Geometry check sheet. Reference: the model listing, model coordinates, mm. A direction names the side the tool comes from. Coordinates: 2 decimals unless noted, no trailing zeros. Order: outer loops, then holes, each group sorted by start corner. A loop starts at its lowest first (then second) coordinate and runs counter-clockwise, first axis right, second up. Notation, with made-up numbers: (52.25, -12) -> (87.25, -12) arc R13 ccw to (87.25, -2) -> close; hole circle Ø10 at (89, 63.25). An arc over 180 degrees is marked (long way). Answer as CSV lines item,"result". Start each with the question number.
from build123d import *

# Parameters (mm, degrees)
F0_R     = 8.5
F1_DEPTH = 4
F2_R     = 5
F3_DEPTH = 100


with BuildPart() as f1:
    # F0 (on Top) → F1 (new body)
    with BuildSketch(Plane.XY):
        Circle(F0_R)
    extrude(amount=F1_DEPTH)

    # F2 (on Top) → F3 (join)
    with BuildSketch(Plane.XY):
        Circle(F2_R)
    extrude(amount=F3_DEPTH)

    # F4 (on Right) → F5 (revolve)
    with BuildSketch(Plane.YZ):
        with BuildLine():
            Line((0, 104.582576), (0, 100))
            Line((0, 100), (5, 100))
            ThreePointArc((5, 100), (4.1833, 102.738613), (2, 104.582576))
            Line((2, 104.582576), (0, 104.582576))
        make_face()
    revolve(axis=Axis((0, 0, 104.791288), (0, 0, -1)))

    # F4 (on Right) → F6 (revolve)
    with BuildSketch(Plane.YZ):
        with BuildLine():
            ThreePointArc((0, 105), (1.021548, 104.894532), (2, 104.582576))
            Line((2, 104.582576), (1, 109.582576))
            Line((1, 109.582576), (0, 109.582576))
            Line((0, 109.582576), (0, 105))
        make_face()
        with BuildLine():
            Line((0, 105), (0, 104.582576))
            Line((0, 104.582576), (2, 104.582576))
            ThreePointArc((2, 104.582576), (1.021548, 104.894532), (0, 105))
        make_face()
    revolve(axis=Axis((0, 0, 104.791288), (0, 0, -1)))


solid = f1.part
Q1. Sectioned sample at B-B, the plane x = 6.25. Record the cut outline in (y, z), then the cut area to 3 significant figures.
Q2. Access from +Z, -Z, +X, -X, +Y, -Y to the whole of each face (thin tool, end or side, straight path). Record for faces 4 (the cylindrical face through (4.57, 7.167, 1.972)), 5 (the flat face through (4, -4, 4)).
Q3. Go/stop test with flat-tipped pins: pin 1 Ø8 at (x, z) = (3.5, 52) entering from +Y; pin 2 Ø10 at (y, z) = (-4.5, 46.5) entering from -X; pin 3 Ø3 at (x, y) = (5.5, 6.5) entering from +Z. Record where each tip stops, or that it passes through.
Q4. Thickness scan on L1, parallel to Z at x = 5.75, y = -5; L2, parallel to Y at x = 0, z = 73.5. Record the ranges inside material, lowest first.
Q5. Sectioned sample at A-A, the plane z = 10. Record the cut outline in (x, y).
Q6. Release check for a two-part mould opening along Z. For faces 1 (the cylindrical face through (-1.08, -4.88, 51.33)), 2 (the flat face through (0, 0, 109.583)), 3 (the flat face through (0, 0, 0)) record: released by +Z, released by -Z, zero draft, split by the parting line, or undercut.
Geometry results:
1,outline,"(-5.76, 0) -> (5.76, 0) -> (5.76, 4) -> (-5.76, 4) -> close"
1,area,"46.1 mm^2"
2,face 4,"+Z, -Z"
2,face 5,"+Z"
3,pin 1,"stops at y = 5"
3,pin 2,"stops at x = -5"
3,pin 3,"stops at z = 4"
4,L1,"z = 0 to 4"
4,L2,"y = -5 to 5"
5,outline,"circle Ø10 at (0, 0)"
6,face 1,"zero draft"
6,face 2,"released by +Z"
6,face 3,"released by -Z"
